from build123d import *

# Parameters (mm, degrees)
SKETCH_1_W               = 50
SKETCH_1_H               = 90
EXTRUDE_1_DEPTH          = 50
SKETCH_2_W               = 25
SKETCH_2_H               = 55.3
CUT_EXTRUDE_1_DEPTH      = 10
SKETCH_3_W               = 85
SKETCH_3_H               = 45
CUT_EXTRUDE_2_DEPTH      = 84.815273071
CUT_EXTRUDE_3_DEPTH      = 106.948100502
CUT_EXTRUDE_3_DEPTH_BACK = 106.948100502


with BuildPart() as part:
    # 草图1 → 凸台-拉伸1 (new body)
    with BuildSketch(Plane(origin=(0, 0, 0), x_dir=(1, 0, 0), z_dir=(0, 1, 0))):
        Rectangle(SKETCH_1_W, SKETCH_1_H)
    extrude(amount=EXTRUDE_1_DEPTH)

    # 草图2 → 切除-拉伸1 (cut)
    with BuildSketch(Plane(origin=(0, 50, 0), x_dir=(1, 0, 0), z_dir=(0, 1, 0))):
        with Locations((-7.5, 11.65)):
            Rectangle(SKETCH_2_W, SKETCH_2_H)
    extrude(amount=-CUT_EXTRUDE_1_DEPTH, mode=Mode.SUBTRACT)

    # 草图3 → 切除-拉伸2 (cut, through all)
    with BuildSketch(Plane.ZY.offset(25)):
        with Locations((0, 25)):
            Rectangle(SKETCH_3_W, SKETCH_3_H)
    extrude(amount=-CUT_EXTRUDE_2_DEPTH, mode=Mode.SUBTRACT)

    # 草图4 → 切除-拉伸3 (cut, two sides: drawn at the far end of the back side and taken through both)
    with BuildSketch(Plane.XY.offset(45).offset(-CUT_EXTRUDE_3_DEPTH_BACK)):
        with BuildLine():
            Line((-11.625, 25), (-11.625, 50))
            Line((-11.625, 50), (-8.375, 50))
            Line((-8.375, 50), (-8.375, 25))
            ThreePointArc((-8.375, 25), (-10, 23.375), (-11.625, 25))
        make_face()
    extrude(amount=CUT_EXTRUDE_3_DEPTH + CUT_EXTRUDE_3_DEPTH_BACK, mode=Mode.SUBTRACT)


solid = part.part
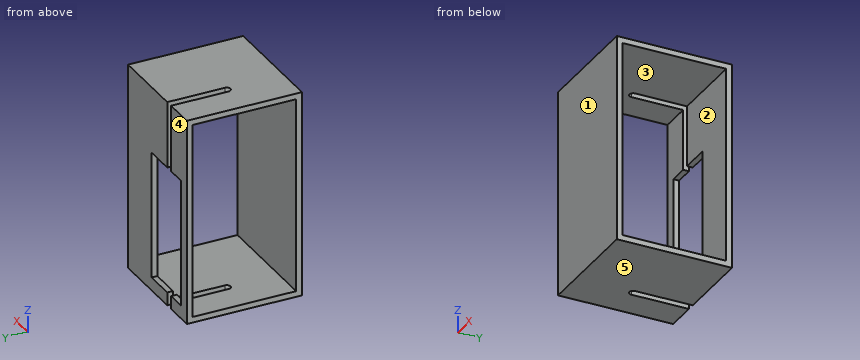
Geometry: final body of the model. Coordinates: model frame, mm. Face numbers are marked on the shaded views. A direction names the side the tool comes from. Give positions to 0.01 mm unless a question says otherwise; leave off trailing zeros. Order: outer loops, then holes, each group sorted by start corner. A loop starts at its lowest first (then second) coordinate and runs counter-clockwise, first axis right, second up. Notation, with made-up numbers: (64.25, 46.5) -> (109.25, 46.5) arc R32 cw to (109.25, 81.5) -> close; hole circle Ø8 at (71, 41.5). An arc over 180 degrees is marked (long way). Write each question's results on one line, items separated by ' | '.
1) Cut plane C-C (x = 11.5). Output: boundary loops of the cut face in (y, z).
Geometry says:
outline: (0, -45) -> (50, -45) -> (50, 45) -> (0, 45) -> close; hole (2.5, -42.5) -> (47.5, -42.5) -> (47.5, 42.5) -> (2.5, 42.5) -> close
2) Cut plane B-B (y = 20). Output: boundary loops of the cut face in (x, z).
Geometry says:
outline: (-25, -45) -> (25, -45) -> (25, -42.5) -> (-25, -42.5) -> close; (-25, 42.5) -> (25, 42.5) -> (25, 45) -> (-25, 45) -> close
3) Set-up query: the marked faces 1 and 2. Return all of +Z, -Z, +X, -X, +Y, -Y with unobstructed straight access to the full face (end or side cutting, diameter ignored); none if empty.
Geometry says:
face 1: +Z, -Z, +X, -X, -Y | face 2: +X, -X
4) Draft query along Y for the marked faces 3, 4 and 5. Return one class per face: released by +Y, released by -Y, zero draft, split by the parting line, or undercut.
Geometry says:
face 3: undercut | face 4: released by +Y | face 5: zero draft
5) Line query: line 1 along Y through (x, z) = (17.5, -22.5); line 2 along Z through (x, y) = (5, 9); line 3 along Y through (x, z) = (-12, -9). Output: solid intervals per line, ascending.
Geometry says:
line 1: y = 0 to 2.5, 47.5 to 50 | line 2: z = -45 to -42.5, 42.5 to 45 | line 3: y = 0 to 2.5
6) Cut plane D-D (y = 43). Output: boundary loops of the cut face in (x, z) (3 decimals), and give its area (3 significant figures).
Geometry says:
outline: (-25, -45) -> (-11.625, -45) -> (-11.625, -42.5) -> (-25, -42.5) -> close; (-25, 42.5) -> (-11.625, 42.5) -> (-11.625, 45) -> (-25, 45) -> close; (-8.375, -45) -> (25, -45) -> (25, -42.5) -> (-8.375, -42.5) -> close; (-8.375, 42.5) -> (25, 42.5) -> (25, 45) -> (-8.375, 45) -> close | area: 234 mm²
7) Cut plane A-A (z = 36). Output: boundary loops of the cut face in (x, y) (3 decimals), and give its area (3 significant figures).
Geometry says:
outline: (-25, 0) -> (25, 0) -> (25, 2.5) -> (-25, 2.5) -> close; (-25, 47.5) -> (-11.625, 47.5) -> (-11.625, 50) -> (-25, 50) -> close; (-8.375, 47.5) -> (25, 47.5) -> (25, 50) -> (-8.375, 50) -> close | area: 242 mm²
8) First-contact query: pin 1 Ø20 at (y, z) = (33.5, 28.5) entering from +X. Flat tip, straight axial feed; report the tip coordinate or a pass-through.
Geometry says:
pin 1: passes through
